Input: part model. Units: mm. Frame: model coordinates. Round coordinates to 2 decimals unless told otherwise and drop trailing zeros. Loops run counter-clockwise (first coordinate to the right, second up) from the corner with the lowest first, then second, coordinate; pieces in that order, holes last. Notation, with made-up numbers: (54.25, 27) -> (61.25, 27) arc R24 ccw to (61.25, 47) -> close; hole circle Ø4 at (48.25, 17.5). An arc over 180 degrees is marked (long way). Answer as a JSON object with one key per item and string values.
```python
from build123d import *

# Parameters (mm, degrees)
SKETCH_1_R          = 1.6
EXTRUDE_1_DEPTH     = 2
FILLET_1_R          = 8
CUT_EXTRUDE_1_DEPTH = 10
FILLET_2_R          = 1


with BuildPart() as part:
    # 草图1 → 凸台-拉伸1 (new body)
    with BuildSketch(Plane.XY):
        Polygon((-30, 0), (30, 0), (50, -40.7), (35, -90), (-35, -90), (-50, -40.7), align=None)
        with Locations((-25, -10)):
            Circle(SKETCH_1_R, mode=Mode.SUBTRACT)
        with Locations((-46, -40.7)):
            Circle(SKETCH_1_R, mode=Mode.SUBTRACT)
        with Locations((25, -10)):
            Circle(SKETCH_1_R, mode=Mode.SUBTRACT)
        with Locations((46, -40.7)):
            Circle(SKETCH_1_R, mode=Mode.SUBTRACT)
        with Locations((-25, -40)):
            Circle(SKETCH_1_R, mode=Mode.SUBTRACT)
        with Locations((25, -40)):
            Circle(SKETCH_1_R, mode=Mode.SUBTRACT)
        with Locations((-25, -70)):
            Circle(SKETCH_1_R, mode=Mode.SUBTRACT)
        with Locations((25, -70)):
            Circle(SKETCH_1_R, mode=Mode.SUBTRACT)
    extrude(amount=EXTRUDE_1_DEPTH)

    # 圆角1
    fillet_1_edges = [part.edges().sort_by_distance(p)[0] for p in [
        (50, -40.7, 1),
        (35, -90, 1),
        (-35, -90, 1),
        (-50, -40.7, 1),
        (-30, 0, 1),
        (30, 0, 1),
    ]]
    fillet(fillet_1_edges, radius=FILLET_1_R)

    # 草图2 → 切除-拉伸1 (cut)
    with BuildSketch(Plane.XY.offset(2)):
        with BuildLine():
            Line((-2.5, -61.668705484), (-2.5, -90))
            Line((-2.5, -90), (2.5, -90))
            Line((2.5, -90), (2.5, -61.668705484))
            ThreePointArc((2.5, -61.668705484), (0, -39.45), (-2.5, -61.668705484))
        make_face()
    extrude(amount=-CUT_EXTRUDE_1_DEPTH, mode=Mode.SUBTRACT)

    # 圆角2
    fillet_2_edges = [part.edges().sort_by_distance(p)[0] for p in [
        (2.5, -61.668705484, 1),
        (-2.5, -61.668705484, 1),
        (-2.5, -90, 1),
        (2.5, -90, 1),
    ]]
    fillet(fillet_2_edges, radius=FILLET_2_R)


solid = part.part
```
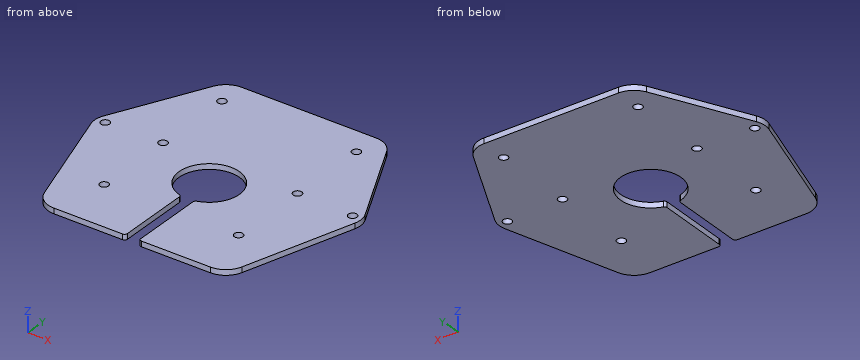
1) Ray query, probe 1 along Y at (x, z) = (-25, 0.5); probe 2 along X at (y, z) = (-70, 1.45); probe 3 along X at (y, z) = (-11, 1.45). Return the intervals inside material, ascending.
Output:
{"probe 1": "y = -90 to -71.6, -68.4 to -41.6, -38.4 to -11.6, -8.4 to 0", "probe 2": "x = -41.09 to -26.6, -23.4 to -2.5, 2.5 to 23.4, 26.6 to 41.09", "probe 3": "x = -35.41 to -26.25, -23.75 to 23.75, 26.25 to 35.41"}
2) Section B-B, the plane y = -54. Output: boundary loops of the cut face in (x, z), plus the area to 3 significant figures.
Output:
{"outline": "(-45.95, 0) -> (-10.76, 0) -> (-10.76, 2) -> (-45.95, 2) -> close; (10.76, 0) -> (45.95, 0) -> (45.95, 2) -> (10.76, 2) -> close", "area": "141 mm^2"}
3) Section D-D, the plane x = 0. Output: boundary loops of the cut face in (y, z), plus the area to 3 significant figures.
Output:
{"outline": "(-39.45, 0) -> (0, 0) -> (0, 2) -> (-39.45, 2) -> close", "area": "78.9 mm^2"}
4) Section C-C, the plane x = 10. Output: boundary loops of the cut face in (y, z), plus the area to 3 significant figures.
Output:
{"outline": "(-90, 0) -> (-55.85, 0) -> (-55.85, 2) -> (-90, 2) -> close; (-45.55, 0) -> (0, 0) -> (0, 2) -> (-45.55, 2) -> close", "area": "159 mm^2"}
5) Contact query for a flat-ended pin moving along its axis: P1, Ø2.5, axis at x = -25, y = -70, coming from the +Z side. Output: stop coordinate, or through.
Output:
{"P1": "passes through"}
6) Section A-A, the plane z = 0.75. Count the separate pieces of the cut face and the enclosed holes in it, plus the area to 3 significant figures.
Output:
{"separate pieces": "1", "enclosed holes": "8", "area": "6,820 mm^2"}
